Check sheet for the drawn part. Datum: minimum x, y, z corner. Units: mm. Give positions to 0.01 mm unless a question says otherwise; leave off trailing zeros. Write each loop counter-clockwise with the first axis right and the second up, starting at its lowest first coordinate (ties: lowest second). Pieces come first, ordered by that corner, then holes. Notation, with made-up numbers: (-40, -17.75) - (-16, -17.75) arc R19 ccw to (-16, -13.75) - close; hole circle Ø2 at (33, -16.5). An arc over 180 degrees is marked (long way). Use a Markdown table: item, result.
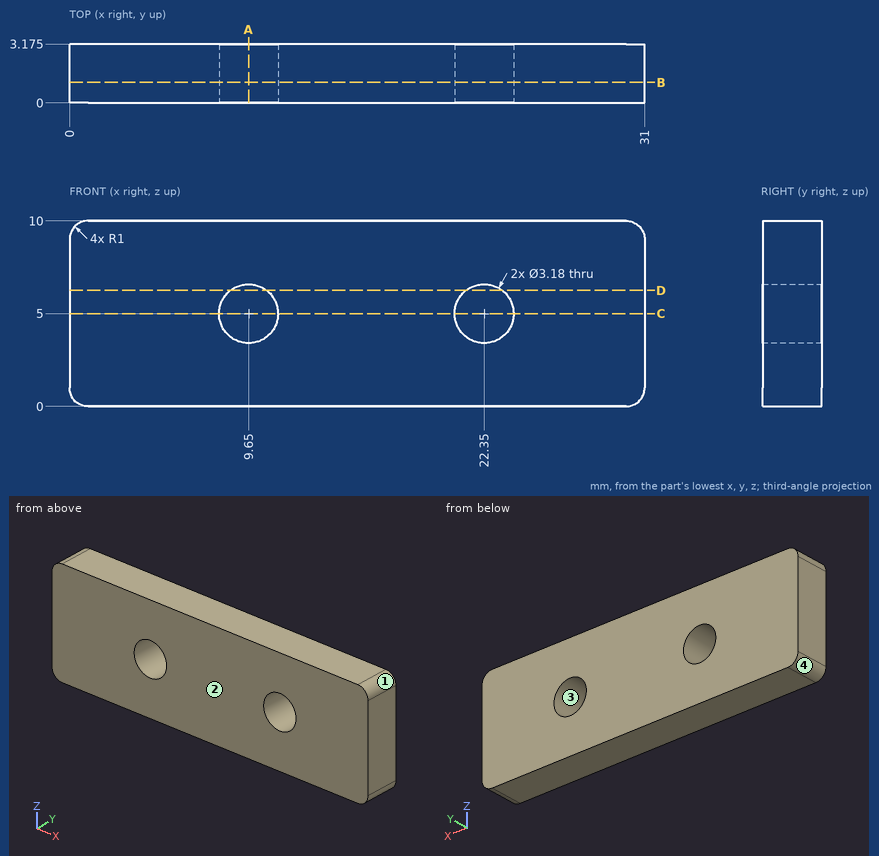
1) Section check C-C on z = 5. Record the boundary of the cut face in (x, y) (3 decimals), then the cut area to 3 significant figures.
Working result:
| item | result |
|---|---|
| outline | (0, 0) - (8.06, 0) - (8.06, 3.175) - (0, 3.175) - close; (11.24, 0) - (20.76, 0) - (20.76, 3.175) - (11.24, 3.175) - close; (23.94, 0) - (31, 0) - (31, 3.175) - (23.94, 3.175) - close |
| area | 78.2 mm² |
2) Mould release check, pull along X, two halves, no side actions. Record for the marked faces 1, 2, 3 and 4: pulls with the +X half, pulls with the -X half, needs draft (parallel to the pull), parting line crosses it, or undercut.
Working result:
| item | result |
|---|---|
| face 1 | pulls with the +X half |
| face 2 | needs draft |
| face 3 | undercut |
| face 4 | pulls with the -X half |
3) Section check A-A on x = 9.65. Record the boundary of the cut face in (y, z) (3 decimals).
Working result:
| item | result |
|---|---|
| outline | (0, 0) - (3.175, 0) - (3.175, 3.41) - (0, 3.41) - close; (0, 6.59) - (3.175, 6.59) - (3.175, 10) - (0, 10) - close |
4) Section check D-D on z = 6.25. Record the boundary of the cut face in (x, y) (3 decimals), then the cut area to 3 significant figures.
Working result:
| item | result |
|---|---|
| outline | (0, 0) - (8.667, 0) - (8.667, 3.175) - (0, 3.175) - close; (10.633, 0) - (21.367, 0) - (21.367, 3.175) - (10.633, 3.175) - close; (23.333, 0) - (31, 0) - (31, 3.175) - (23.333, 3.175) - close |
| area | 85.9 mm² |
5) Section check B-B on y = 1.1. Record the boundary of the cut face in (x, z).
Working result:
| item | result |
|---|---|
| outline | (0, 1) arc R1 ccw to (1, 0) - (30, 0) arc R1 ccw to (31, 1) - (31, 9) arc R1 ccw to (30, 10) - (1, 10) arc R1 ccw to (0, 9) - close; hole circle Ø3.18 at (9.65, 5); hole circle Ø3.18 at (22.35, 5) |
6) Material ranges on L1, parallel to X at y = 2.3, z = 5; L2, parallel to X at y = 2.6, z = 6; L3, parallel to Z at x = 9, y = 1.65, recorded low to high. Write a range as from..to.
Working result:
| item | result |
|---|---|
| L1 | x = 0..8.06, 11.24..20.76, 23.94..31 |
| L2 | x = 0..8.41, 10.89..21.11, 23.59..31 |
| L3 | z = 0..3.55, 6.45..10 |
